Check sheet for the modelled part. Datum: model origin and axes. Units: mm. Round coordinates to 2 decimals unless told otherwise and drop trailing zeros. Write each loop counter-clockwise with the first axis right and the second up, starting at its lowest first coordinate (ties: lowest second). Pieces come first, ordered by that corner, then holes. Notation, with made-up numbers: (-13, 41) -> (17, 41) arc R10 ccw to (17, 47) -> close; hole circle Ø3 at (-23, 41). An arc over 180 degrees is marked (long way). Write item = value, one per line.
from build123d import *

# Parameters (mm, degrees)
BOSS_EXTRUDE1_DEPTH       = 5
M6_CLEARANCE_HOLE1_D      = 6.6
M6_CLEARANCE_HOLE1_DEPTH  = 6
M6_CLEARANCE_HOLE1_TIP    = 1.982840043
LPATTERN1_COUNT           = 13
LPATTERN1_PITCH           = 40
LPATTERN2_COUNT           = 12
LPATTERN2_PITCH           = 40
M25_CLEARANCE_HOLE1_D     = 27
M25_CLEARANCE_HOLE1_DEPTH = 6
M25_CLEARANCE_HOLE1_TIP   = 8.111618357


with BuildPart() as part:
    # Sketch1 → Boss-Extrude1 (new body)
    with BuildSketch(Plane.XY):
        with BuildLine():
            Line((-270, -60), (270, -60))
            ThreePointArc((270, -60), (277.071067812, -57.071067812), (280, -50))
            Line((280, -50), (280, 50))
            ThreePointArc((280, 50), (277.071067812, 57.071067812), (270, 60))
            Line((270, 60), (-270, 60))
            ThreePointArc((-270, 60), (-277.071067812, 57.071067812), (-280, 50))
            Line((-280, 50), (-280, -50))
            ThreePointArc((-280, -50), (-277.071067812, -57.071067812), (-270, -60))
        make_face()
    extrude(amount=BOSS_EXTRUDE1_DEPTH)

    # M6 Clearance Hole1
    with Locations(Plane.XY.offset(5)):
        with Locations((270, 0), (-270, 0)):
            Hole(M6_CLEARANCE_HOLE1_D / 2, depth=M6_CLEARANCE_HOLE1_DEPTH)
            with Locations((0, 0, -(M6_CLEARANCE_HOLE1_DEPTH + M6_CLEARANCE_HOLE1_TIP / 2))):  # 118° drill point
                Cone(0, M6_CLEARANCE_HOLE1_D / 2, M6_CLEARANCE_HOLE1_TIP, mode=Mode.SUBTRACT)

    # Sketch4 → M20 Clearance Hole1 (revolve, cut)
    with BuildSketch(Plane(origin=(240, -30, 0), x_dir=(0, 1, 0), z_dir=(1, 0, 0))):
        Polygon((0, 0), (0, 12.609466809), (11, 6), (11, 0), align=None)
    m20_clearance_hole1 = revolve(axis=Axis((240, -30, -6.35), (0, 0, 1)), mode=Mode.SUBTRACT)

    # LPattern1: M20 Clearance Hole1 ×13
    with Locations(*[(-i * LPATTERN1_PITCH, 0, 0) for i in range(1, LPATTERN1_COUNT)]):
        add(m20_clearance_hole1, mode=Mode.SUBTRACT)

    # Sketch6 → M22 Clearance Hole1 (revolve, cut)
    with BuildSketch(Plane(origin=(224, 15, 0), x_dir=(0, 1, 0), z_dir=(1, 0, 0))):
        Polygon((0, 0), (0, 13.210327428), (12, 6), (12, 0), align=None)
    m22_clearance_hole1 = revolve(axis=Axis((224, 15, -6.35), (0, 0, 1)), mode=Mode.SUBTRACT)

    # LPattern2: M22 Clearance Hole1 ×12
    with Locations(*[(-i * LPATTERN2_PITCH, 0, 0) for i in range(1, LPATTERN2_COUNT)]):
        add(m22_clearance_hole1, mode=Mode.SUBTRACT)

    # M25 Clearance Hole1
    with Locations(Plane(origin=(0, 0, 0), x_dir=(-1, 0, 0), z_dir=(0, 0, -1))):
        with Locations((216, 15)):
            Hole(M25_CLEARANCE_HOLE1_D / 2, depth=M25_CLEARANCE_HOLE1_DEPTH)
            with Locations((0, 0, -(M25_CLEARANCE_HOLE1_DEPTH + M25_CLEARANCE_HOLE1_TIP / 2))):  # 118° drill point
                Cone(0, M25_CLEARANCE_HOLE1_D / 2, M25_CLEARANCE_HOLE1_TIP, mode=Mode.SUBTRACT)


solid = part.part
(1) Release check for a two-part mould opening along X. For faces 1 (the cylindrical face through (-276.99, 57.15, 2.46)), 2 (the cylindrical face through (-50.906, -31.432, 2.465)) record: pulls with the +X half, pulls with the -X half, needs draft (parallel to the pull), parting line crosses it, or undercut.
Worked answers:
face_1 = pulls with the -X half
face_2 = undercut
(2) Material ranges on L1, parallel to Y at x = -161, z = 1.4; L2, parallel to Y at x = -23, z = 2.7; L3, parallel to Y at x = 74.5, z = 4.2, recorded low to high. Write a range as [from, to].
Worked answers:
L1 = [-60, -40.95], [-19.05, 60]
L2 = [-60, 5.25], [24.75, 60]
L3 = [-60, -39.53], [-20.47, 9.19], [20.81, 60]
(3) Sectioned sample at D-D on x = 64. Enter the section's corners in (y, z).
Worked answers:
outline = (-60, 0) -> (3, 0) -> (3, 5) -> (-60, 5) -> close; (27, 0) -> (60, 0) -> (60, 5) -> (27, 5) -> close
(4) Sectioned sample at B-B on y = -30. Count the separate pieces of the cut face and the enclosed holes in it, then the cut area to 3 significant figures.
Worked answers:
separate_pieces = 14
enclosed_holes = 0
area = 1,370 mm²
(5) Go/stop test with a flat-tipped pin: P1, Ø21.5, axis at x = -96, y = 15, coming from the +Z side. Record where the tip stops, or that it passes through.
Worked answers:
P1 = through
(6) Sectioned sample at A-A on x = -216. Enter the section's corners in (y, z), then the cut area to 3 significant figures.
Worked answers:
outline = (-60, 0) -> (1.5, 0) -> (1.5, 5) -> (-60, 5) -> close; (28.5, 0) -> (60, 0) -> (60, 5) -> (28.5, 5) -> close
area = 465 mm²
